from build123d import *

# Parameters (mm, degrees)
F0_W      = 70
F0_H      = 50
F1_DEPTH  = 10
F2_W      = 51.701616
F2_H      = 40.25942
F3_DEPTH  = 20
F5_DEPTH  = 2.2
F6_R      = 2.5
F7_DEPTH  = 42.93071
F9_DEPTH  = 3
F10_R     = 2.5
F11_DEPTH = 42.13071
F12_W     = 101.047278
F12_H     = 53.498119
F13_DEPTH = 30.001


with BuildPart() as f1:
    # F0 (on Top) → F1 (new body)
    with BuildSketch(Plane.XY):
        Rectangle(F0_W, F0_H)
    extrude(amount=F1_DEPTH)

    # F2 (on face) → F3 (join)
    with BuildSketch(Plane.XY.offset(10)):
        Rectangle(F2_W, F2_H)
    extrude(amount=F3_DEPTH)

    # F4 (on face) → F5 (cut)
    with BuildSketch(Plane.XZ.offset(20.12971)):
        Polygon((-9.302341, 18.084529), (-9.302341, 22.703331), (-13.302341, 25.012733), (-17.302341, 22.703331), (-17.302341, 18.084529), (-13.302341, 15.775128), align=None)
    extrude(amount=-F5_DEPTH, mode=Mode.SUBTRACT)

    # F6 (on face) → F7 (cut, through all)
    with BuildSketch(Plane.XZ.offset(17.92971)):
        with Locations((-13.302341, 20.39393)):
            Circle(F6_R)
    extrude(amount=-F7_DEPTH, mode=Mode.SUBTRACT)

    # F8 (on face) → F9 (cut)
    with BuildSketch(Plane.XZ.offset(20.12971)):
        Polygon((16.465587, 17.672712), (16.465587, 23.446215), (11.465587, 26.332966), (6.465587, 23.446215), (6.465587, 17.672712), (11.465587, 14.785961), align=None)
    extrude(amount=-F9_DEPTH, mode=Mode.SUBTRACT)

    # F10 (on face) → F11 (cut, through all)
    with BuildSketch(Plane.XZ.offset(17.12971)):
        with Locations((11.465587, 20.559464)):
            Circle(F10_R)
    extrude(amount=-F11_DEPTH, mode=Mode.SUBTRACT)

    # F12 (on Top) → F13 (cut, through all)
    with BuildSketch(Plane.XY):
        with Locations((0, 26.749059)):
            Rectangle(F12_W, F12_H)
    extrude(amount=F13_DEPTH, mode=Mode.SUBTRACT)


solid = f1.part
Check sheet for the modelled part. Datum: model origin and axes. Units: mm. A direction names the side the tool comes from. Coordinates: 2 decimals unless noted, no trailing zeros. Write each loop counter-clockwise with the first axis right and the second up, starting at its lowest first coordinate (ties: lowest second). Pieces come first, ordered by that corner, then holes. Notation, with made-up numbers: M -4,23.5 L 5,23.5 A15 cw 5,49.5 Z; hole C 65.25,64 d11. An arc over 180 degrees is marked long. Answer as CSV lines item,"result".
Q1. Material ranges on probe 1 along X at (y, z) = (-5, 22.5); probe 2 along Y at (x, z) = (1.5, 17.75); probe 3 along X at (y, z) = (-9.25, 27.25), recorded low to high. Write a range as from..to.
Check result:
probe 1,"-25.85..-14.65, -11.96..9.89, 13.04..25.85"
probe 2,"-20.13..0"
probe 3,"-25.85..25.85"
Q2. Set-up check for faces 1 (the face through (25.851, -10, 20)), 2 (the face through (-25.851, -10, 20)), 3 (the face through (-17.302, -19, 20)): record each of +Z, -Z, +X, -X, +Y, -Y from which the full face is reachable in a straight line by a thin tool's end or side.
Check result:
face 1,"+Z, +X, +Y, -Y"
face 2,"+Z, -X, +Y, -Y"
face 3,"-Y"
Q3. Cross-section at C-C (z = 11.75). Record the boundary of the cut face in (x, y), then the cut area to 3 significant figures.
Check result:
outline,"M -25.85,-20.13 L 25.85,-20.13 L 25.85,0 L -25.85,0 Z"
area,"1,040 mm^2"
Q4. Cross-section at B-B (x = -2.5). Record the boundary of the cut face in (y, z), then the cut area to 3 significant figures.
Check result:
outline,"M -25,0 L 0,0 L 0,30 L -20.13,30 L -20.13,10 L -25,10 Z"
area,"653 mm^2"
Q5. Cross-section at A-A (y = -5.5). Record the boundary of the cut face in (x, z), then the cut area to 3 significant figures.
Check result:
outline,"M -35,0 L 35,0 L 35,10 L 25.85,10 L 25.85,30 L -25.85,30 L -25.85,10 L -35,10 Z; hole C -13.3,20.39 d5; hole C 11.47,20.56 d5"
area,"1,690 mm^2"
Q6. Go/stop test with flat-tipped pins: pin 1 (0.9 mm diameter, centred on y = -19, z = 20.5, fed in from +X); pin 2 (6.5 mm diameter, centred on x = 11.47, z = 20.56, fed in from -Y); pin 3 (10 mm diameter, centred on y = -15, z = 20, fed in from -X). Record where each tip stops, or that it passes through.
Check result:
pin 1,"x = 25.85"
pin 2,"y = -17.13"
pin 3,"x = -25.85"
Q7. Cross-section at D-D (x = -28.5). Record the boundary of the cut face in (y, z).
Check result:
outline,"M -25,0 L 0,0 L 0,10 L -25,10 Z"
